Input: part model. Units: mm. Frame: model coordinates. Coordinates: 2 decimals unless noted, no trailing zeros. Order: outer loops, then holes, each group sorted by start corner. A loop starts at its lowest first (then second) coordinate and runs counter-clockwise, first axis right, second up.
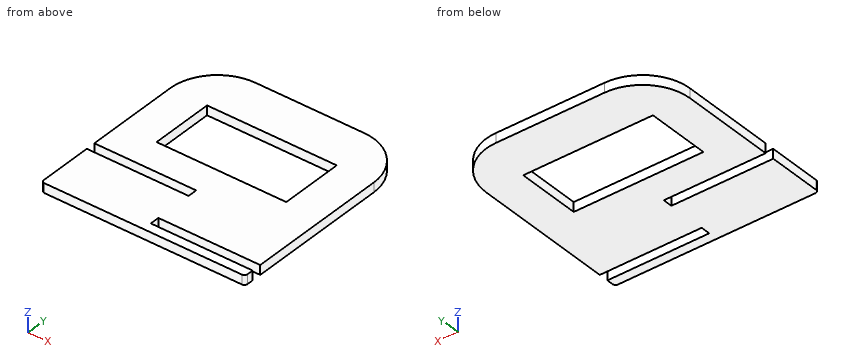
from build123d import *

# Parameters (mm, degrees)
SKETCH1_W           = 41
SKETCH1_H           = 20
BOSS_EXTRUDE7_DEPTH = 3


with BuildPart() as part:
    # Sketch1 → Boss-Extrude7 (new body)
    with BuildSketch(Plane.XY):
        with BuildLine():
            Line((-49.661503554, -6.420867766), (-15.261503554, -6.420867766))
            ThreePointArc((-15.261503554, -6.420867766), (-4.654901836, -10.814266048), (-0.261503554, -21.420867766))
            Line((-0.261503554, -21.420867766), (-0.261503554, -66.420867766))
            Line((-0.261503554, -66.420867766), (-32.461503554, -66.420867766))
            Line((-32.461503554, -66.420867766), (-32.461503554, -69.420867766))
            Line((-32.461503554, -69.420867766), (-0.261503554, -69.420867766))
            Line((-0.261503554, -69.420867766), (-0.261503554, -71.420867766))
            ThreePointArc((-0.261503554, -71.420867766), (-0.554396773, -72.127974547), (-1.261503554, -72.420867766))
            Line((-1.261503554, -72.420867766), (-63.661503554, -72.420867766))
            ThreePointArc((-63.661503554, -72.420867766), (-64.368610335, -72.127974547), (-64.661503554, -71.420867766))
            Line((-64.661503554, -71.420867766), (-64.661503554, -54.420867766))
            Line((-64.661503554, -54.420867766), (-32.461503554, -54.420867766))
            Line((-32.461503554, -54.420867766), (-32.461503554, -51.420867766))
            Line((-32.461503554, -51.420867766), (-64.661503554, -51.420867766))
            Line((-64.661503554, -51.420867766), (-64.661503554, -21.420867766))
            ThreePointArc((-64.661503554, -21.420867766), (-60.268105272, -10.814266048), (-49.661503554, -6.420867766))
        make_face()
        with Locations((-32.461503554, -31.420867766)):
            Rectangle(SKETCH1_W, SKETCH1_H, mode=Mode.SUBTRACT)
    extrude(amount=BOSS_EXTRUDE7_DEPTH)


solid = part.part
Item 1: Pin query (flat end, axial travel): pin 1 Ø1.5 at (y, z) = (-68, 2) entering from +X; pin 2 Ø1.5 at (x, z) = (-53.5, 2) entering from +Y; pin 3 Ø1.5 at (y, z) = (-53, 1) entering from -X. Return the tip coordinate at first contact, or that it passes through.
Response values:
pin 1: stops at x = -32.46
pin 2: stops at y = -6.74
pin 3: stops at x = -32.46
Item 2: Cut plane B-B on x = -23. Return loops of the section in (y, z).
Response values:
outline: (-72.42, 0) - (-69.42, 0) - (-69.42, 3) - (-72.42, 3) - close; (-66.42, 0) - (-41.42, 0) - (-41.42, 3) - (-66.42, 3) - close; (-21.42, 0) - (-6.42, 0) - (-6.42, 3) - (-21.42, 3) - close
Item 3: Cut plane A-A on y = -30. Return loops of the section in (x, z), then the cut area to 3 significant figures.
Response values:
outline: (-64.66, 0) - (-52.96, 0) - (-52.96, 3) - (-64.66, 3) - close; (-11.96, 0) - (-0.26, 0) - (-0.26, 3) - (-11.96, 3) - close
area: 70.2 mm2
Item 4: Ray query, probe 1 along Y at (x, z) = (-45, 1.5); probe 2 along Y at (x, z) = (-28.5, 1.25); probe 3 along X at (y, z) = (-35, 1.5). Return the intervals inside material, ascending.
Response values:
probe 1: y = -72.42 to -54.42, -51.42 to -41.42, -21.42 to -6.42
probe 2: y = -72.42 to -69.42, -66.42 to -41.42, -21.42 to -6.42
probe 3: x = -64.66 to -52.96, -11.96 to -0.26
Item 5: Cut plane D-D on x = -10. Return loops of the section in (y, z), then the cut area to 3 significant figures.
Response values:
outline: (-72.42, 0) - (-69.42, 0) - (-69.42, 3) - (-72.42, 3) - close; (-66.42, 0) - (-7.37, 0) - (-7.37, 3) - (-66.42, 3) - close
area: 186 mm2
Item 6: Cut plane C-C on z = 0.55. Return loops of the section in (x, y), then the cut area to 3 significant figures.
Response values:
outline: (-64.66, -71.42) arc R1 ccw to (-63.66, -72.42) - (-1.26, -72.42) arc R1 ccw to (-0.26, -71.42) - (-0.26, -69.42) - (-32.46, -69.42) - (-32.46, -66.42) - (-0.26, -66.42) - (-0.26, -21.42) arc R15 ccw to (-15.26, -6.42) - (-49.66, -6.42) arc R15 ccw to (-64.66, -21.42) - (-64.66, -51.42) - (-32.46, -51.42) - (-32.46, -54.42) - (-64.66, -54.42) - close; hole (-52.96, -41.42) - (-11.96, -41.42) - (-11.96, -21.42) - (-52.96, -21.42) - close
area: 3,140 mm2
